from build123d import *

# Parameters (mm, degrees)
BOSS_EXTRUDE1_DEPTH = 25.4
SKETCH2_R           = 3
CUT_EXTRUDE1_DEPTH  = 28.944
CHAMFER1_SIZE       = 3.3
FILLET1_R           = 2


with BuildPart() as part:
    # Sketch1 → Boss-Extrude1 (new body)
    with BuildSketch(Plane(origin=(0, 0, 0), x_dir=(0, 0, -1), z_dir=(1, 0, 0))):
        Polygon((-0.970833333, 15.458470238), (-11.892833333, 15.458470238), (-11.892833333, -20.863529762), (16.051166667, -20.863529762), (16.051166667, 28.158470238), (5.129166667, 28.158470238), (5.129166667, -9.941529762), (-0.970833333, -9.941529762), align=None)
    extrude(amount=BOSS_EXTRUDE1_DEPTH)

    # Sketch2 → Cut-Extrude1 (cut, through all)
    with BuildSketch(Plane(origin=(0, 0, -16.051166667), x_dir=(-1, 0, 0), z_dir=(0, 0, -1))):
        with Locations((-12.7, 21.658470238)):
            Circle(SKETCH2_R)
        with Locations((-12.7, -14.363529762)):
            Circle(SKETCH2_R)
    extrude(amount=-CUT_EXTRUDE1_DEPTH, mode=Mode.SUBTRACT)

    # Chamfer1
    chamfer1_edges = [part.edges().sort_by_distance(p)[0] for p in [
        (15.7, 21.658470238, -5.129166667),
        (15.7, -14.363529762, 11.892833333),
    ]]
    chamfer(chamfer1_edges, length=CHAMFER1_SIZE)

    # Fillet1
    fillet1_edges = [part.edges().sort_by_distance(p)[0] for p in [
        (12.7, 15.458470238, 11.892833333),
        (12.7, 15.458470238, 0.970833333),
        (25.4, 15.458470238, 6.431833333),
        (0, 15.458470238, 6.431833333),
    ]]
    fillet(fillet1_edges, radius=FILLET1_R)


solid = part.part
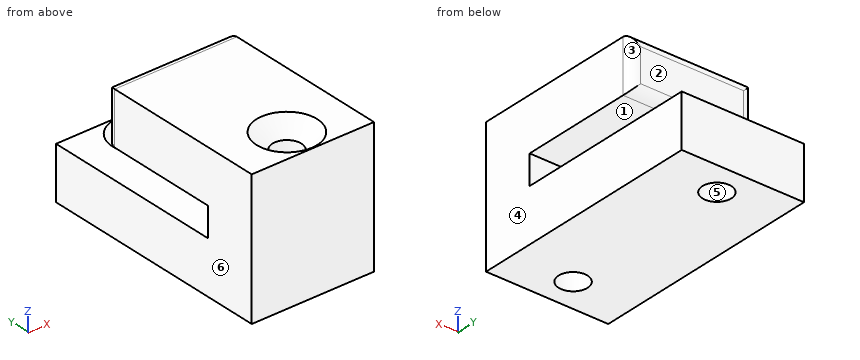
Work out the finished part from the listing and answer in its coordinate system (mm). Face numbers are marked on the shaded views. A direction names the side the tool comes from. Give positions to 0.01 mm unless a question says otherwise; leave off trailing zeros. Order: outer loops, then holes, each group sorted by start corner. A loop starts at its lowest first (then second) coordinate and runs counter-clockwise, first axis right, second up. Notation, with made-up numbers: (-27.75, -32) -> (5.25, -32) arc R31 cw to (5.25, 4) -> close; hole circle Ø4 at (10.25, -15.5). An arc over 180 degrees is marked (long way). Answer as a JSON object with one key per item and string values. Group by question number.
1. Section B-B on y = -1.5 is taken. Determine the outline of the cut face in (x, z), plus the area to 3 significant figures.
2. Consider line 1 along Y through (x, z) = (12.7, -11.5); line 2 along Y through (x, z) = (12.7, -4.25); line 3 along Z through (x, y) = (16.5, 6.5). Determine where each line is inside the solid, lowest interval first. Write a range as [from, to].
3. Section C-C on x = 3 is taken. Determine the outline of the cut face in (y, z), plus the area to 3 significant figures.
4. The mould has two halves that part along X. Classify the marked faces 4, 5 and 6: released by +X, released by -X, zero draft, split by the parting line, or undercut.
5. Section A-A on x = 12.7 is taken. Determine the outline of the cut face in (y, z).
6. Flat-ended cylindrical pins translate along their axes: pin 1 Ø7 at (x, y) = (12.7, 21.66) entering from +Z; pin 2 Ø5.5 at (x, z) = (13, 8) entering from +Y; pin 3 Ø1.8 at (x, z) = (16, -3) entering from +Y. Find the tip coordinate at first contact, or state that the pin passes through.
7. Section D-D on z = 5 is taken. Determine the outline of the cut face in (x, y), plus the area to 3 significant figures.
8. A tool of negligible diameter and unlimited length cuts with its end or side. For the marked faces 1, 2 and 3, from which of +Z, -Z, +X, -X, +Y, -Y can it reach the whole face along a straight path? Write none if from no direction.
Result sheet:
{
 "1": {"outline": "(0, -16.05) -> (25.4, -16.05) -> (25.4, -5.13) -> (0, -5.13) -> close; (0, 0.97) -> (25.4, 0.97) -> (25.4, 11.89) -> (0, 11.89) -> close", "area": "555 mm^2"},
 "2": {"line 1": "y = [-20.86, -17.36], [-11.36, 18.66], [24.66, 28.16]", "line 2": "y = [-20.86, -17.36], [-11.36, -9.94]", "line 3": "z = [-16.05, -5.13], [0.97, 11.89]"},
 "3": {"outline": "(-20.86, -16.05) -> (28.16, -16.05) -> (28.16, -5.13) -> (-9.94, -5.13) -> (-9.94, 0.97) -> (13.46, 0.97) arc R2 ccw to (15.46, 2.97) -> (15.46, 9.89) arc R2 ccw to (13.46, 11.89) -> (-20.86, 11.89) -> close", "area": "997 mm^2"},
 "4": {"face 4": "released by +X", "face 5": "undercut", "face 6": "released by -X"},
 "5": {"outline": "(-20.86, -16.05) -> (-17.36, -16.05) -> (-17.36, 8.59) -> (-20.66, 11.89) -> (-20.86, 11.89) -> close; (-11.36, -16.05) -> (18.66, -16.05) -> (18.66, -8.43) -> (15.36, -5.13) -> (-9.94, -5.13) -> (-9.94, 0.97) -> (13.46, 0.97) arc R2 ccw to (15.46, 2.97) -> (15.46, 9.89) arc R2 ccw to (13.46, 11.89) -> (-8.06, 11.89) -> (-11.36, 8.59) -> close; (24.66, -16.05) -> (28.16, -16.05) -> (28.16, -5.13) -> (27.96, -5.13) -> (24.66, -8.43) -> close"},
 "6": {"pin 1": "stops at z = -7.93", "pin 2": "stops at y = 15.46", "pin 3": "stops at y = -9.94"},
 "7": {"outline": "(0, -20.86) -> (25.4, -20.86) -> (25.4, 13.46) arc R2 ccw to (23.4, 15.46) -> (2, 15.46) arc R2 ccw to (0, 13.46) -> close; hole circle Ø6 at (12.7, -14.36)", "area": "893 mm^2"},
 "8": {"face 1": "+X, -X, +Y", "face 2": "+Z, +X, -X, +Y", "face 3": "+Z, +X, +Y"}
}
